from build123d import *

# Parameters (mm, degrees)
CUT_EXTRUDE1_REACH             = 162.072
SKETCH2_W                      = 4
SKETCH2_H                      = 1
CUT_EXTRUDE1_DIRECTION_2_REACH = 162.072


with BuildPart() as part:
    # Sketch1 → Revolve1 (revolve)
    with BuildSketch(Plane(origin=(0, 0, 0), x_dir=(1, 0, 0), z_dir=(0, 1, 0)), mode=Mode.PRIVATE) as revolve1_sk:
        Polygon((0, 2.4), (0, 2.1), (-6, 2.1), (-6, 0), (160, 0), (160, 2.1), (154.5, 2.1), (154.5, 2.4), (138.3, 2.4), (138.3, 3.1), (109.9, 3.1), (109.9, 3.4), (7.5, 3.4), (7.5, 2.4), align=None)
    revolve(revolve1_sk.sketch.rotate(Axis((-12.266501292, 0, 0), (1, 0, 0)), 180), axis=Axis((-12.266501292, 0, 0), (1, 0, 0)))

    # Sketch2 → Cut-Extrude1 (cut, up to next)
    with BuildSketch(Plane(origin=(0, 0, 0), x_dir=(1, 0, 0), z_dir=(0, 1, 0)), mode=Mode.PRIVATE) as cut_extrude1_sk1:
        with Locations((9.5, 2.9)):
            Rectangle(SKETCH2_W, SKETCH2_H)
    cut_extrude1_tool1 = extrude(cut_extrude1_sk1.sketch, amount=-CUT_EXTRUDE1_REACH, mode=Mode.PRIVATE) & part.part
    # Sketch2 → Cut-Extrude1 (cut, up to next)
    with BuildSketch(Plane(origin=(0, 0, 0), x_dir=(1, 0, 0), z_dir=(0, 1, 0)), mode=Mode.PRIVATE) as cut_extrude1_sk2:
        with Locations((9.5, -2.9)):
            Rectangle(SKETCH2_W, SKETCH2_H)
    cut_extrude1_tool2 = extrude(cut_extrude1_sk2.sketch, amount=-CUT_EXTRUDE1_REACH, mode=Mode.PRIVATE) & part.part
    add(cut_extrude1_tool1.solids().sort_by_distance((9.5, 0, -2.9))[0], mode=Mode.SUBTRACT)
    add(cut_extrude1_tool2.solids().sort_by_distance((9.5, 0, 2.9))[0], mode=Mode.SUBTRACT)

    # Sketch2 → Cut-Extrude1 direction 2 (cut, up to next)
    with BuildSketch(Plane(origin=(0, 0, 0), x_dir=(1, 0, 0), z_dir=(0, 1, 0)), mode=Mode.PRIVATE) as cut_extrude1_direction_2_sk1:
        with Locations((9.5, 2.9)):
            Rectangle(SKETCH2_W, SKETCH2_H)
    cut_extrude1_direction_2_tool1 = extrude(cut_extrude1_direction_2_sk1.sketch, amount=CUT_EXTRUDE1_DIRECTION_2_REACH, mode=Mode.PRIVATE) & part.part
    # Sketch2 → Cut-Extrude1 direction 2 (cut, up to next)
    with BuildSketch(Plane(origin=(0, 0, 0), x_dir=(1, 0, 0), z_dir=(0, 1, 0)), mode=Mode.PRIVATE) as cut_extrude1_direction_2_sk2:
        with Locations((9.5, -2.9)):
            Rectangle(SKETCH2_W, SKETCH2_H)
    cut_extrude1_direction_2_tool2 = extrude(cut_extrude1_direction_2_sk2.sketch, amount=CUT_EXTRUDE1_DIRECTION_2_REACH, mode=Mode.PRIVATE) & part.part
    add(cut_extrude1_direction_2_tool1.solids().sort_by_distance((9.5, 0, -2.9))[0], mode=Mode.SUBTRACT)
    add(cut_extrude1_direction_2_tool2.solids().sort_by_distance((9.5, 0, 2.9))[0], mode=Mode.SUBTRACT)


solid = part.part
Can you work these out from the model? Positions are in its coordinate system, mm. A direction names the side the tool comes from. Round coordinates to 2 decimals unless told otherwise and drop trailing zeros. Loops run counter-clockwise (first coordinate to the right, second up) from the corner with the lowest first, then second, coordinate; pieces in that order, holes last. Notation, with made-up numbers: (38, 78) - (81, 78) arc R28 cw to (81, 117) - close; hole circle Ø4 at (26.5, 80.5). An arc over 180 degrees is marked (long way). Write item = value, one per line. Start each with the question number.
(1) If we section it at B-B (x = 118): Please give me the cut outline in (y, z).
(2) If we section it at A-A (z = 0): Please give me the cut outline in (x, y), and give its area (3 significant figures).
(3) For P1, Ø3, axis at x = 23, y = 2.5, coming from the +Z side; P2, Ø1, axis at x = 126.5, z = -2, coming from the -Y side; P3, Ø3, axis at x = 9.5, y = 0.5, coming from the +Z side, each with a flat end and sliding along its axis, tell me the tip position at first contact or that it passes through.
(4) For faces 1 (the face through (138.3, 2, -2)), 2 (the face through (-3.042, -0.631, 2.003)), 3 (the face through (9, 0, -2.4)), which set-ups out of +Z, -Z, +X, -X, +Y, -Y let a thin tool reach every point of the face, with its end or its side?
(5) If I drill on probe 1 along X at (y, z) = (-1, 3); probe 2 along Z at (x, y) = (82.5, -0.25); probe 3 along X at (y, z) = (-1.5, -2.5), over which ranges is the centre line in solid material (lowest first)? Write a range as [from, to].
(6) If we section it at C-C (x = 75): Please give me the cut outline in (y, z).
Ans:
q1.outline = circle Ø6.2 at (0, 0)
q2.outline = (-6, -2.1) - (0, -2.1) - (0, -2.4) - (7.5, -2.4) - (7.5, -3.4) - (109.9, -3.4) - (109.9, -3.1) - (138.3, -3.1) - (138.3, -2.4) - (154.5, -2.4) - (154.5, -2.1) - (160, -2.1) - (160, 2.1) - (154.5, 2.1) - (154.5, 2.4) - (138.3, 2.4) - (138.3, 3.1) - (109.9, 3.1) - (109.9, 3.4) - (7.5, 3.4) - (7.5, 2.4) - (0, 2.4) - (0, 2.1) - (-6, 2.1) - close
q2.area = 1,030 mm²
q3.P1 = 3.25
q3.P2 = -2.71
q3.P3 = 2.4
q4.face_1 = +X
q4.face_2 = -X
q4.face_3 = -Z, -X, +Y, -Y
q5.probe_1 = [11.5, 109.9]
q5.probe_2 = [-3.39, 3.39]
q5.probe_3 = [11.5, 138.3]
q6.outline = circle Ø6.8 at (0, 0)
